The drawing under review shows one solid part. Ordinate dimensions are in mm from its lowest x, y, z. A direction names the side the tool comes from. Coordinates: 2 decimals unless noted, no trailing zeros. Order: outer loops, then holes, each group sorted by start corner. A loop starts at its lowest first (then second) coordinate and runs counter-clockwise, first axis right, second up. Notation, with made-up numbers: M 12,18 L 67,18 A13 cw 67,42 Z; hole C 13,38.25 d7. An arc over 180 degrees is marked long. Answer as a JSON object with one key per item and string values.
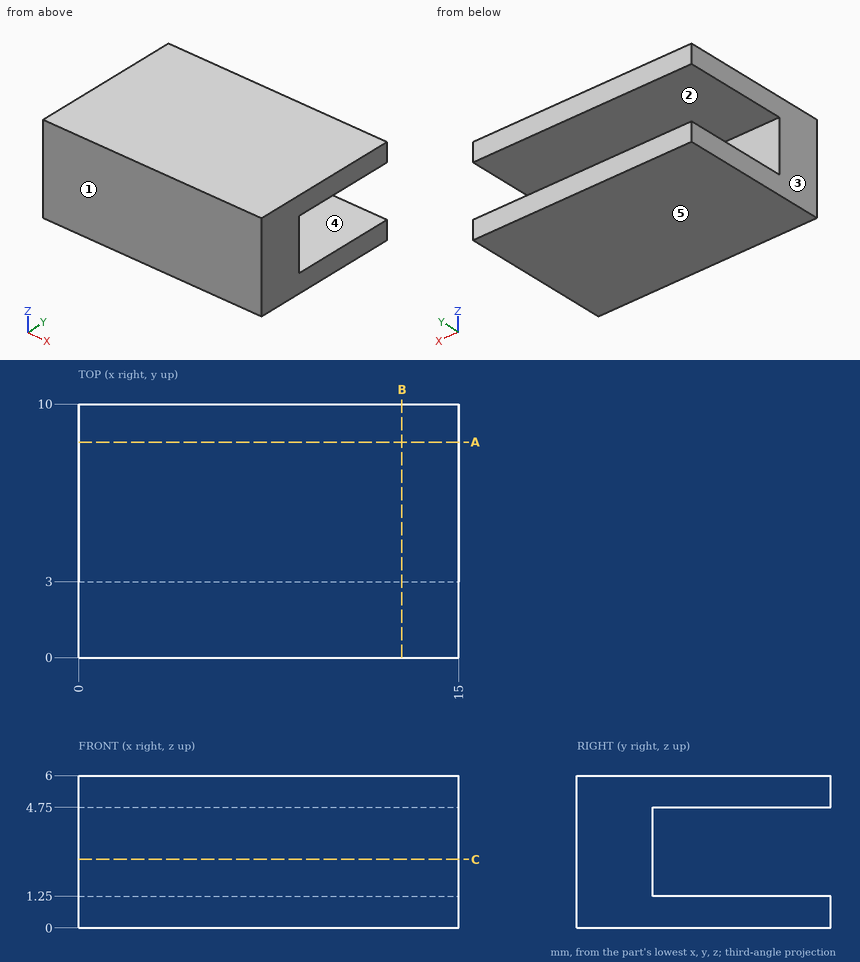
1) Mouldability with a two-part tool opening along Z and no side actions: class the marked faces 3, 4 and 5 as released by +Z, released by -Z, zero draft, split by the parting line, or undercut.
Taken from the geometry:
{"face 3": "zero draft", "face 4": "undercut", "face 5": "released by -Z"}
2) To check wall thickness, follow L1, parallel to Z at x = 2.75, y = 7.5; L2, parallel to Y at x = 14, z = 1.4. State the ranges of each line that lie inside material, in increasing order.
Taken from the geometry:
{"L1": "z = 0 to 1.25, 4.75 to 6", "L2": "y = 0 to 3"}
3) Add section C-C (z = 2.7). State the section outline as (x, y) points, and give its area (3 significant figures).
Taken from the geometry:
{"outline": "M 0,0 L 15,0 L 15,3 L 0,3 Z", "area": "45.0 mm2"}
4) Insertion check: pin 1 Ø2 at (y, z) = (6, 2.5) entering from +X; pin 2 Ø1.8 at (x, z) = (8.5, 3.5) entering from +Y. Each pin has a flat end and moves straight along its axis. Give the tip position at first contact, or say it passes through.
Taken from the geometry:
{"pin 1": "passes through", "pin 2": "stops at y = 3"}
5) Add section B-B (x = 12.75). State the section outline as (y, z) points, and give its area (3 significant figures).
Taken from the geometry:
{"outline": "M 0,0 L 10,0 L 10,1.25 L 3,1.25 L 3,4.75 L 10,4.75 L 10,6 L 0,6 Z", "area": "35.5 mm2"}
6) Tool access review of the marked faces 1 and 2: name each direction out of +Z, -Z, +X, -X, +Y, -Y from which nothing blocks a thin tool from reaching the whole face with its end or side.
Taken from the geometry:
{"face 1": "+Z, -Z, +X, -X, -Y", "face 2": "+X, -X, +Y"}
7) Add section A-A (y = 8.5). State the section outline as (x, z) points, and give its area (3 significant figures).
Taken from the geometry:
{"outline": "M 0,0 L 15,0 L 15,1.25 L 0,1.25 Z; M 0,4.75 L 15,4.75 L 15,6 L 0,6 Z", "area": "37.5 mm2"}
